Input: part model. Units: mm. Frame: model coordinates. Face numbers are marked on the shaded views. A direction names the side the tool comes from. Coordinates: 2 decimals unless noted, no trailing zeros. Loops run counter-clockwise (first coordinate to the right, second up) from the corner with the lowest first, then second, coordinate; pieces in that order, holes last.
Item 1: Section D-D on x = -14. Return loops of the section in (y, z), and give its area (3 significant figures).
Item 2: Section B-B on y = 9. Return loops of the section in (x, z) (3 decimals), and give its area (3 significant figures).
Item 3: Section C-C on z = 11. Return loops of the section in (x, y).
Item 4: Ray query, line 1 along Z through (x, y) = (10, 13); line 2 along Y through (x, z) = (2.5, 33.5); line 3 along X through (y, z) = (2.75, 15). Return the intervals inside material, ascending.
Item 5: Reachability of the marked faces 1, 2, 3, 4 and 5 from +Z, -Z, +X, -X, +Y, -Y: full face, straight path, thin tool, end or side. Return the list, or none.
Item 6: Contact query for flat-ended pins moving along their axis: P1, Ø9, axis at x = 8.5, y = 7, coming from the +Z side; P2, Ø2, axis at x = -5.5, z = 32.5, coming from the +Y side; P3, Ø8, axis at y = 7, z = 17.5, coming from the +X side. Output: stop coordinate, or through.
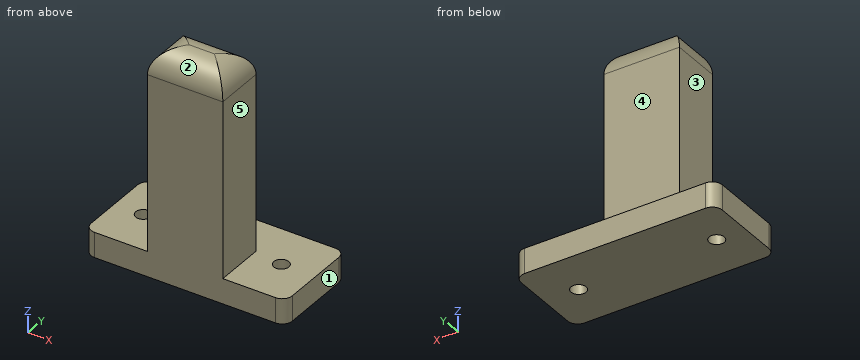
```python
from build123d import *

# Parameters (mm, degrees)
F0_W     = 40
F0_H     = 18
F1_DEPTH = 5
F2_W     = 15
F2_H     = 10
F3_DEPTH = 40
F4_R     = 4.99999
F5_D     = 3
F5_DEPTH = 50
F5_TIP   = 0.9012909285
F6_R     = 2


# Not quite as in the source:
# - a fillet or chamfer is up to 0.001 mm smaller than in the source, because OpenCascade refuses the exact size


with BuildPart() as f1:
    # F0 (on Top) → F1 (new body)
    with BuildSketch(Plane.XY):
        with Locations((-0.0778210488, 9)):
            Rectangle(F0_W, F0_H)
    extrude(amount=F1_DEPTH)

    # F2 (on face) → F3 (join)
    with BuildSketch(Plane.XY.offset(5)):
        with Locations((-0.0778210488, 5)):
            Rectangle(F2_W, F2_H)
    extrude(amount=F3_DEPTH)

    # F4 (radius 5 in the source; OpenCascade refuses exactly that, so slightly less here)
    f4_edges = [f1.edges().sort_by_distance(p)[0] for p in [
        (7.422179, 5, 45),
        (-0.077821, 10, 45),
        (-7.577821, 5, 45),
        (-0.077821, 0, 45),
    ]]
    fillet(f4_edges, radius=F4_R)

    # F5
    with Locations(Plane.XY.offset(5)):
        with Locations((-14.3456859514, 9), (13.1249977276, 9)):
            Hole(F5_D / 2, depth=F5_DEPTH)
            with Locations((0, 0, -(F5_DEPTH + F5_TIP / 2))):  # 118° drill point
                Cone(0, F5_D / 2, F5_TIP, mode=Mode.SUBTRACT)

    # F6
    f6_edges = [f1.edges().sort_by_distance(p)[0] for p in [
        (-20.077821, 0, 2.5),
        (-20.077821, 18, 2.5),
        (19.922179, 18, 2.5),
        (19.922179, 0, 2.5),
    ]]
    fillet(f6_edges, radius=F6_R)


solid = f1.part
```
Results found:
1. outline: (0, 0) - (7.54, 0) - (7.54, 5) - (0, 5) - close; (10.46, 0) - (18, 0) - (18, 5) - (10.46, 5) - close
1. area: 75.4 mm2
2. outline: (-20.078, 0) - (-15.846, 0) - (-15.846, 5) - (-20.078, 5) - close; (-12.846, 0) - (11.625, 0) - (11.625, 5) - (7.422, 5) - (7.422, 40) arc R5 ccw to (6.422, 43) - (-6.578, 43) arc R5 ccw to (-7.578, 40) - (-7.578, 5) - (-12.846, 5) - close; (14.625, 0) - (19.922, 0) - (19.922, 5) - (14.625, 5) - close
2. area: 738 mm2
3. outline: (-7.58, 0) - (7.42, 0) - (7.42, 10) - (-7.58, 10) - close
4. line 1: z = 0 to 5
4. line 2: y = 0 to 10
4. line 3: x = -7.58 to 7.42
5. face 1: +Z, -Z, +X, +Y, -Y
5. face 2: +Z, +X, -X, -Y
5. face 3: +Z, -X, +Y, -Y
5. face 4: +Z, +X, -X, +Y
5. face 5: +Z, +X, +Y, -Y
6. P1: stops at z = 44.74
6. P2: stops at y = 10
6. P3: stops at x = 7.42
